```python
from build123d import *

# Parameters (mm, degrees)
SKETCH4_R           = 4.699
SKETCH4_R_2         = 1.5875
BOSS_EXTRUDE1_DEPTH = 12.7
CUT_EXTRUDE3_DEPTH  = 3.175
CUT_EXTRUDE2_START  = -6.35
CUT_EXTRUDE2_DEPTH  = 6.35
FILLET1_1_64_R      = 0.396875
CHAMFER1_SIZE       = 0.254


with BuildPart() as part:
    # Sketch4 → Boss-Extrude1 (new body)
    with BuildSketch(Plane(origin=(0, 0, 0), x_dir=(1, 0, 0), z_dir=(0, 1, 0))):
        Circle(SKETCH4_R)
        Circle(SKETCH4_R_2, mode=Mode.SUBTRACT)
    extrude(amount=BOSS_EXTRUDE1_DEPTH)

    # Sketch7 → Cut-Extrude3 (cut)
    with BuildSketch(Plane.XZ):
        Polygon((1.649778394, 2.8575), (-1.649778394, 2.8575), (-3.299556788, 0), (-1.649778394, -2.8575), (1.649778394, -2.8575), (3.299556788, 0), align=None)
    extrude(amount=-CUT_EXTRUDE3_DEPTH, mode=Mode.SUBTRACT)

    # Sketch6 → Cut-Extrude2 (cut)
    with BuildSketch(Plane(origin=(0, 12.7, 0), x_dir=(1, 0, 0), z_dir=(0, 1, 0)).offset(CUT_EXTRUDE2_START)):
        Polygon((1.833087105, 3.175), (-1.833087105, 3.175), (-3.666174209, 0), (-1.833087105, -3.175), (1.833087105, -3.175), (3.666174209, 0), align=None)
    extrude(amount=CUT_EXTRUDE2_DEPTH, mode=Mode.SUBTRACT)

    # Fillet1-1/64
    fillet1_1_64_edges = [part.edges().sort_by_distance(p)[0] for p in [
        (2.474667591, 3.175, 1.42875),
        (1.649778394, 1.5875, 2.8575),
        (2.474667591, 3.175, -1.42875),
        (3.299556788, 1.5875, 0),
        (0, 3.175, -2.8575),
        (1.649778394, 1.5875, -2.8575),
        (-2.474667591, 3.175, -1.42875),
        (-1.649778394, 1.5875, -2.8575),
        (-2.474667591, 3.175, 1.42875),
        (-3.299556788, 1.5875, 0),
        (0, 3.175, 2.8575),
        (-1.649778394, 1.5875, 2.8575),
        (0, 6.35, -3.175),
        (-1.833087105, 9.525, -3.175),
        (-2.749630657, 6.35, -1.5875),
        (-3.666174209, 9.525, 0),
        (-2.749630657, 6.35, 1.5875),
        (-1.833087105, 9.525, 3.175),
        (0, 6.35, 3.175),
        (1.833087105, 9.525, 3.175),
        (2.749630657, 6.35, 1.5875),
        (3.666174209, 9.525, 0),
        (2.749630657, 6.35, -1.5875),
        (1.833087105, 9.525, -3.175),
    ]]
    fillet(fillet1_1_64_edges, radius=FILLET1_1_64_R)

    # Chamfer1
    chamfer1_edges = [part.edges().sort_by_distance(p)[0] for p in [
        (-1.5875, 3.175, 0),
        (-4.699, 0, 0),
        (-1.5875, 6.35, 0),
        (-4.699, 12.7, 0),
        (-2.749630657, 12.7, 1.5875),
        (0, 12.7, 3.175),
        (2.749630657, 12.7, 1.5875),
        (2.749630657, 12.7, -1.5875),
        (0, 12.7, -3.175),
        (-2.749630657, 12.7, -1.5875),
        (0, 0, 2.8575),
        (-2.474667591, 0, 1.42875),
        (-2.474667591, 0, -1.42875),
        (0, 0, -2.8575),
        (2.474667591, 0, -1.42875),
        (2.474667591, 0, 1.42875),
        (-3.604777433, 12.7, 0),
        (-1.802388717, 12.7, 3.121828832),
        (1.802388717, 12.7, 3.121828832),
        (3.604777433, 12.7, 0),
        (1.802388717, 12.7, -3.121828832),
        (-1.802388717, 12.7, -3.121828832),
        (-1.619080006, 0, 2.804328832),
        (-3.238160012, 0, 0),
        (-1.619080006, 0, -2.804328832),
        (1.619080006, 0, -2.804328832),
        (3.238160012, 0, 0),
        (1.619080006, 0, 2.804328832),
    ]]
    chamfer(chamfer1_edges, length=CHAMFER1_SIZE)


solid = part.part
```
Model file for the job. Use its own axes, mm. A direction names the side the tool comes from. Give positions to 0.01 mm unless a question says otherwise; leave off trailing zeros. Loops run counter-clockwise (first coordinate to the right, second up) from the corner with the lowest first, then second, coordinate; pieces in that order, holes last. Notation, with made-up numbers: M -10,44.25 L 6,44.25 A20 cw 6,53.25 Z; hole C 77.25,44 d3. An arc over 180 degrees is marked long. Use one line per item in the form item = value.
Item 1: Drill centre lines: L1, parallel to X at y = 11, z = 0; L2, parallel to Z at x = 0, y = 5.2; L3, parallel to X at y = 3, z = -2. Where is each one in solid material? Low to high.
Filled in:
L1 = -4.7 to -3.6, 3.6 to 4.7
L2 = -4.7 to -1.59, 1.59 to 4.7
L3 = -4.25 to -2.07, 2.07 to 4.25
Item 2: Which spindle directions (+Z, -Z, +X, -X, +Y, -Y) get a long thin tool onto all of the face, cutting with end or side? Do faces 4 (the flat face through (2.87, 12.57, -1.63)), 5 (the flat face through (-2.465, 1.498, 1.446)), 6 (the flat face through (-3, 12.7, -2)). Say none if no direction does.
Filled in:
face_4 = +Y
face_5 = -Y
face_6 = +Z, -Z, +X, -X, +Y
Item 3: Slice it at B-B on y = 8.25. List the corners of the cut face in (x, z) (3 decimals).
Filled in:
outline = C 0,0 d9.398; hole M -3.552,-0.198 L -1.948,-2.977 A0.397 ccw -1.604,-3.175 L 1.604,-3.175 A0.397 ccw 1.948,-2.977 L 3.552,-0.198 A0.397 ccw 3.552,0.198 L 1.948,2.977 A0.397 ccw 1.604,3.175 L -1.604,3.175 A0.397 ccw -1.948,2.977 L -3.552,0.198 A0.397 ccw Z
Item 4: Flat gauge pins, fed straight in: pin 1 Ø1.6 at (x, y) = (-1, 11) entering from -Z; pin 2 Ø3 at (y, z) = (3, -2) entering from -X; pin 3 Ø4 at (x, y) = (-3.5, 5) entering from +Z; pin 4 Ø1 at (x, y) = (0.5, 9) entering from +Z. Where does each tip first touch, or does it go through?
Filled in:
pin_1 = -4.69
pin_2 = -4.67
pin_3 = 4.45
pin_4 = 4.7
Item 5: Two-plate mould, pull along Z, no slides. Class faces 1 (the flat face through (2.57, 0.13, -1.51)), 2 (the cylindrical face through (-0.61, 6.26, -4.66)), 3 (the flat face through (-3, 0, 2)): released by +Z, released by -Z, zero draft, split by the parting line, or undercut.
Filled in:
face_1 = undercut
face_2 = split by the parting line
face_3 = zero draft
Item 6: Slice it at C-C on y = 4.75. List the corners of the cut face in (x, z) (1 decimal).
Filled in:
outline = C 0,0 d9.4; hole C 0,0 d3.2
